Geometry: see drawing. Coordinates: mm, zero at the bounding-box minimum. Round coordinates to 2 decimals unless told otherwise and drop trailing zeros. Order: outer loops, then holes, each group sorted by start corner. A loop starts at its lowest first (then second) coordinate and runs counter-clockwise, first axis right, second up. Notation, with made-up numbers: (30.25, -33) -> (48.25, -33) arc R29 cw to (48.25, -5) -> close; hole circle Ø7 at (35.5, 30). An arc over 180 degrees is marked (long way). Put each result on its own line as item: value.
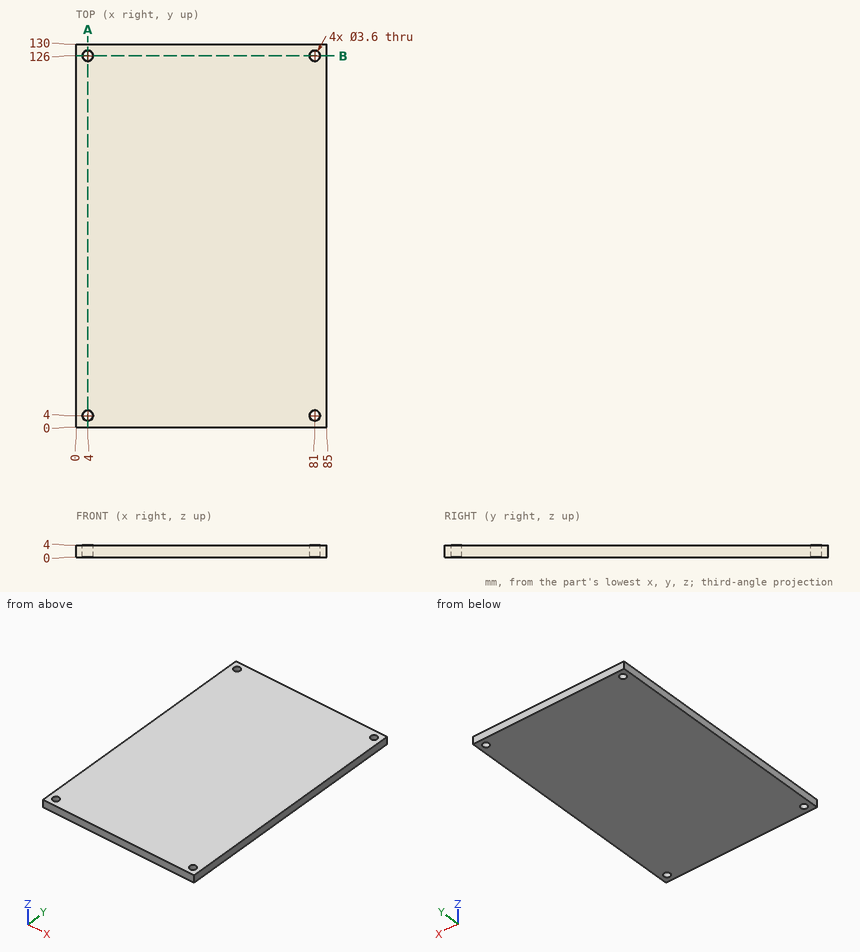
1. Cut plane A-A on x = 4. Return loops of the section in (y, z).
Ans:
outline: (0, 0) -> (2.2, 0) -> (2.2, 4) -> (0, 4) -> close; (5.8, 0) -> (124.2, 0) -> (124.2, 4) -> (5.8, 4) -> close; (127.8, 0) -> (130, 0) -> (130, 4) -> (127.8, 4) -> close
2. Cut plane B-B on y = 126. Return loops of the section in (x, z).
Ans:
outline: (0, 0) -> (2.2, 0) -> (2.2, 4) -> (0, 4) -> close; (5.8, 0) -> (79.2, 0) -> (79.2, 4) -> (5.8, 4) -> close; (82.8, 0) -> (85, 0) -> (85, 4) -> (82.8, 4) -> close
3. Material intervals for probe 1 along X at (y, z) = (126, 2.15); probe 2 along Y at (x, z) = (81, 2.3), sorted ascending.
Ans:
probe 1: 0 to 2.2, 5.8 to 79.2, 82.8 to 85
probe 2: 0 to 2.2, 5.8 to 124.2, 127.8 to 130
4. Contact query for flat-ended pins moving along their axis: P1, Ø3, axis at x = 4, y = 4, coming from the +Z side; P2, Ø12, axis at x = 44.5, y = 100, coming from the -Z side. Output: stop coordinate, or through.
Ans:
P1: through
P2: z = 0
